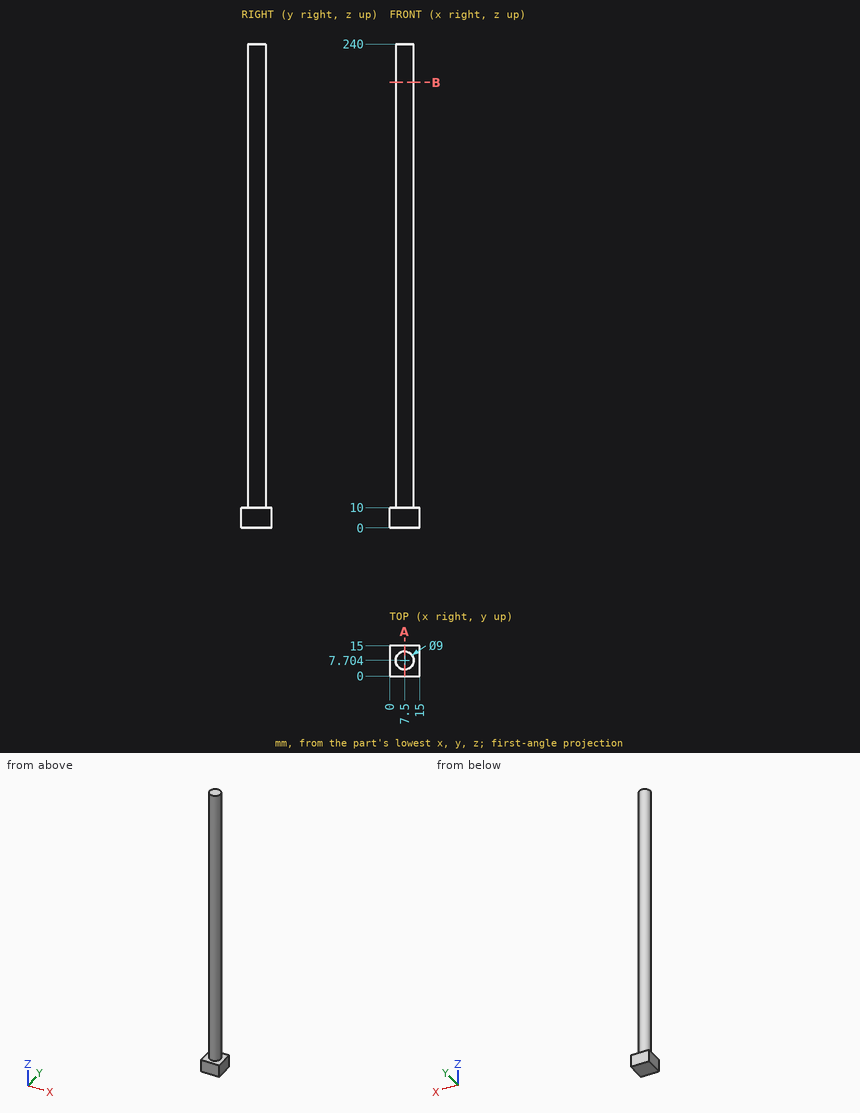
Study the drawing (mm; zero at the part's minimum x, y, z) and answer. Coordinates: 2 decimals unless noted, no trailing zeros. Order: outer loops, then holes, each group sorted by start corner. A loop starts at its lowest first (then second) coordinate and runs counter-clockwise, first axis right, second up. Notation, with made-up numbers: (68.25, -26.75) -> (85.25, -26.75) arc R16 ccw to (85.25, 4.25) -> close; hole circle Ø7 at (-11.5, 76). An arc over 180 degrees is marked (long way). Answer in a Markdown table with one row per item. Add a question column.
Item 1: Find the intervals of material crossed by L1, parallel to Z at x = 11.25, y = 14; L2, parallel to Y at x = 7.5, z = 91.5 (1 decimal); L3, parallel to X at y = 8, z = 127.5, in increasing order. Write a range as from..to.
Item 2: Find section A-A (x = 7.5). Write down the section's boundary in (y, z) (1 decimal), then the cut area to 3 significant figures.
Item 3: Each of these flat-tipped pins is pushed along its axis until it touches: P1, Ø6, axis at x = 4, z = 187, coming from the -Y side; P2, Ø2, axis at x = 4.5, z = 64, coming from the +Y side (1 decimal); P3, Ø1, axis at x = 9, z = 165, coming from the -Y side. Where does it stop, or does it pass through?
Item 4: Find section B-B (z = 221). Write down the section's boundary in (x, y) (1 decimal), then the cut area to 3 significant figures.
Result set:
| question | item | result |
|---|---|---|
| 1 | L1 | z = 0..10 |
| 1 | L2 | y = 3.2..12.2 |
| 1 | L3 | x = 3.01..11.99 |
| 2 | outline | (0, 0) -> (15, 0) -> (15, 10) -> (12.2, 10) -> (12.2, 240) -> (3.2, 240) -> (3.2, 10) -> (0, 10) -> close |
| 2 | area | 2,220 mm² |
| 3 | P1 | stops at y = 3.23 |
| 3 | P2 | stops at y = 11.7 |
| 3 | P3 | stops at y = 3.32 |
| 4 | outline | circle Ø9 at (7.5, 7.7) |
| 4 | area | 63.6 mm² |
